The listing builds one solid part. Answer for the finished solid, in the listing's coordinates (mm). A direction names the side the tool comes from. Round coordinates to 2 decimals unless told otherwise and drop trailing zeros.
(1) For faces 4 (the face through (78.426, -54.965, 0.207)), 5 (the face through (-81.574, 0.207, 2.465)), 6 (the face through (27, 52.5, 0)), determine the directions among +Z, -Z, +X, -X, +Y, -Y from which every point of the face is accessible in a straight line to the end or side of a thin tool.
(2) This flat-tipped pin is pushed along its axis until it touches: pin 1 Ø1.6 at (x, y) = (-80.5, -37.5) entering from +Z. Where does it stop, or does it pass through?
(3) Find the intervals of material crossed by probe 1 along X at (y, z) = (0, 3.3); probe 2 along X at (y, z) = (53.85, 0); probe 3 along Y at (x, z) = (80, 2.35), in increasing order.
(4) The mould has two halves that part along Y. Classify faces 1 (the face through (27, -52.5, 0)), 2 (the face through (-1, 1, -5)), 3 (the face through (-80.477, -39.014, 2.465)): +Y half, -Y half, draft (parallel to the pull), parting line (faces both ways), or undercut.
Autodesk Inventor part; units mm, degrees
ref_plane "YZ Plane" through (0, 0, 0) normal (1, 0, 0) x (0, 1, 0)
ref_plane "XZ Plane" through (0, 0, 0) normal (0, 1, 0) x (-1, 0, 0)
ref_plane "XY Plane" through (0, 0, 0) normal (0, 0, 1) x (1, 0, 0)
sketch "Sketch1" plane through (0, 0, 0) normal (0, 0, 1) x (1, 0, 0)
  line L0 (-85, 57.5) -> (85, 57.5)
  line L1 (85, 57.5) -> (85, -57.5)
  line L2 (85, -57.5) -> (-85, -57.5)
  line L3 (-85, -57.5) -> (-85, 57.5)
  line L4 (-85, 57.5) -> (85, -57.5) construction
  line L5 (85, 57.5) -> (-85, -57.5) construction
  point P0 (0, 0)
  dimension "d0" = 170
  dimension "d1" = 115
extrude "Extrusion1" add sketch "Sketch1" along normal mid plane 10
sketch "Sketch2" plane through (0, 0, 5) normal (0, 0, 1) x (1, 0, 0)
  line L0 (-85, 57.5) -> (-85, -57.5)
  line L1 (-85, -57.5) -> (85, -57.5)
  point P0 (0, 0)
  point P1 (-80, -37.5)
  point P2 (80, -37.5)
  point P3 (-80, 0)
  point P4 (80, 0)
  point P5 (80, 37.5)
  point P6 (-80, 37.5)
  dimension "d4" = 5
  dimension "d5" = 20
  dimension "d11" = 160
  dimension "d55" = 37.5
  dimension "d62" = 37.5
hole "Hole1" at (-80, -37.5, 5) at (-80, 0, 5) at (80, 0, 5) at (80, -37.5, 5) at (-80, 37.5, 5) at (80, 37.5, 5) direction (0, 0, -1) diameter 3.175 depth 5
sketch "Sketch3" plane through (-85, -57.5, 5) normal (0, -1, 0) x (1, 0, 0)
  line L0 (0, 0) -> (0, -10)
  line L1 (0, 0) -> (170, 0)
  point P0 (85, -5)
  point P1 (5, -5)
  point P2 (58.3333, -5)
  point P3 (111.6667, -5)
  point P4 (165, -5)
  dimension "d21" = 5
  dimension "d22" = 5
  dimension "d25" = 53.3333
hole "Hole2" at (-80, -57.5, 0) at (-26.6667, -57.5, 0) at (26.6667, -57.5, 0) at (80, -57.5, 0) direction (0, 1, 0) diameter 3.175 depth 5
sketch "Sketch4" plane through (-85, 57.5, 5) normal (0, 1, 0) x (1, 0, 0)
  line L0 (0, 10) -> (0, 0)
  line L1 (170, 0) -> (0, 0)
  line L2 (0, 10) -> (170, 10)
  point P0 (85, 5)
  point P1 (112.5, 5)
  point P2 (57.5, 5)
  dimension "d67" = 5
  dimension "d69" = 27.5
  dimension "d72" = 55
hole "Hole3" at (27.5, 57.5, 0) at (-27.5, 57.5, 0) direction (0, -1, 0) diameter 3.175 depth 5
properties part number "back"
Solutions:
1. face 4: -Y
1. face 5: +Z
1. face 6: +Y
2. pin 1: stops at z = 0
3. probe 1: x = -85 to -81.59, -78.41 to 78.41, 81.59 to 85
3. probe 2: x = -85 to -29.09, -25.91 to 25.91, 29.09 to 85
3. probe 3: y = -57.5 to -39.09, -35.91 to -1.59, 1.59 to 35.91, 39.09 to 57.5
4. face 1: -Y half
4. face 2: draft
4. face 3: undercut
